Verification items for the finished model (mm, model axes). A direction names the side the tool comes from. Give positions to 0.01 mm unless a question says otherwise; leave off trailing zeros. Write each loop counter-clockwise with the first axis right and the second up, starting at its lowest first coordinate (ties: lowest second). Pieces come first, ordered by that corner, then holes. Notation, with made-up numbers: (-7.75, 63.25) -> (5.25, 63.25) arc R32 ccw to (5.25, 92.25) -> close; hole circle Ø3 at (35, 62). An arc over 180 degrees is marked (long way). Answer as CSV lines item,"result".
```python
from build123d import *

# Parameters (mm, degrees)
F0_W           = 40
F0_H           = 25
F1_DEPTH       = 5
F2_W           = 35
F2_H           = 3
F3_DEPTH       = 25
F4_SIZE        = 0.2
F7_D           = 2.5
F7_CBORE_D     = 3.2
F7_CBORE_DEPTH = 1
F8_D           = 2.5
F8_CBORE_D     = 3.2
F8_CBORE_DEPTH = 1


with BuildPart() as f1:
    # F0 (on Top) → F1 (new body)
    with BuildSketch(Plane.XY):
        with Locations((20, 12.5)):
            Rectangle(F0_W, F0_H)
    extrude(amount=F1_DEPTH)

    # F2 (on face) → F3 (cut)
    with BuildSketch(Plane.XZ):
        with Locations((22.5, 3.5)):
            Rectangle(F2_W, F2_H)
    extrude(amount=-F3_DEPTH, mode=Mode.SUBTRACT)

    # F4
    f4_edges = [f1.edges().sort_by_distance(p)[0] for p in [
        (2.5, 25, 5),
        (5, 12.5, 5),
        (2.5, 0, 5),
        (0, 12.5, 5),
        (20, 0, 0),
        (40, 0, 1),
        (22.5, 0, 2),
        (5, 0, 3.5),
        (0, 0, 2.5),
        (20, 25, 0),
        (0, 25, 2.5),
        (5, 25, 3.5),
        (22.5, 25, 2),
        (40, 25, 1),
    ]]
    chamfer(f4_edges, length=F4_SIZE)

    # F7 (through all)
    with Locations(Plane.XY.offset(5)):
        with Locations((2.6, 20.8)):
            CounterBoreHole(F7_D / 2, F7_CBORE_D / 2, F7_CBORE_DEPTH)

    # F8 (through all)
    with Locations(Plane.XY.offset(5)):
        with Locations((2.6, 4.2)):
            CounterBoreHole(F8_D / 2, F8_CBORE_D / 2, F8_CBORE_DEPTH)


solid = f1.part
```
1) Section check B-B (z = 3.2). Record the boundary of the cut face in (x, y), and give its area (3 significant figures).
Reported:
outline,"(0, 0.2) -> (0.2, 0) -> (4.8, 0) -> (5, 0.2) -> (5, 24.8) -> (4.8, 25) -> (0.2, 25) -> (0, 24.8) -> close; hole circle Ø2.5 at (2.6, 4.2); hole circle Ø2.5 at (2.6, 20.8)"
area,"115 mm²"
2) Section check D-D (x = 23). Record the boundary of the cut face in (y, z).
Reported:
outline,"(0, 0.2) -> (0.2, 0) -> (24.8, 0) -> (25, 0.2) -> (25, 1.8) -> (24.8, 2) -> (0.2, 2) -> (0, 1.8) -> close"
3) Depth check by flat-ended pin: pin 1 (0.8 mm diameter, centred on y = 12.5, z = 3, fed in from +X). Enter the tip coordinate at first touch or a pass-through.
Reported:
pin 1,"x = 5"
4) Draft check along X on faces 4 (the flat face through (0, 12, 2)), 5 (the cylindrical face through (2.392, 5.786, 4.507)), 6 (the flat face through (15, 0, 1)), 7 (the cylindrical face through (2.87, 19.58, 1.97)). Enter one of: +X half, -X half, draft (parallel to the pull), parting line (faces both ways), or undercut.
Reported:
face 4,"-X half"
face 5,"undercut"
face 6,"draft"
face 7,"undercut"
5) Section check A-A (x = 2.6). Record the boundary of the cut face in (y, z), and give its area (3 significant figures).
Reported:
outline,"(0, 0.2) -> (0.2, 0) -> (2.95, 0) -> (2.95, 4) -> (2.6, 4) -> (2.6, 5) -> (0.2, 5) -> (0, 4.8) -> close; (5.45, 0) -> (19.55, 0) -> (19.55, 4) -> (19.2, 4) -> (19.2, 5) -> (5.8, 5) -> (5.8, 4) -> (5.45, 4) -> close; (22.05, 0) -> (24.8, 0) -> (25, 0.2) -> (25, 4.8) -> (24.8, 5) -> (22.4, 5) -> (22.4, 4) -> (22.05, 4) -> close"
area,"98.5 mm²"
6) Tool access check on faces 1 (the flat face through (5, 12, 3)), 2 (the flat face through (15, 25, 1)), 3 (the cylindrical face through (4.126, 21.281, 4.507)). Record the directions out of +Z, -Z, +X, -X, +Y, -Y that give a thin tool (end or side, any length) a straight path to the whole face; none if there is none.
Reported:
face 1,"+Z, +X, +Y, -Y"
face 2,"+Z, -Z, +X, -X, +Y"
face 3,"+Z"
7) Scan lines: line 1 along Y through (x, z) = (2.6, 4.6); line 2 along Y through (x, z) = (2.6, 1.5); line 3 along X through (y, z) = (2.25, 4.55). Record each from-to range of solid material in increasing order.
Reported:
line 1,"0 to 2.6, 5.8 to 19.2, 22.4 to 25"
line 2,"0 to 2.95, 5.45 to 19.55, 22.05 to 25"
line 3,"0 to 5"
8) Section check C-C (y = 20.8). Record the boundary of the cut face in (x, z).
Reported:
outline,"(0, 0) -> (1.35, 0) -> (1.35, 4) -> (1, 4) -> (1, 5) -> (0.2, 5) -> (0, 4.8) -> close; (3.85, 0) -> (40, 0) -> (40, 2) -> (5, 2) -> (5, 4.8) -> (4.8, 5) -> (4.2, 5) -> (4.2, 4) -> (3.85, 4) -> close"
